from build123d import *

# Parameters (mm, degrees)
TUBE_R            = 6.5
TUBE_R_2          = 4.5
TUBE_DEPTH        = 1
PAD001_DEPTH      = 12
CYLINDER018_R     = 4.5
CYLINDER018_DEPTH = 500
CYLINDER012_R     = 11.5
CYLINDER012_DEPTH = 1
PAD_DEPTH         = 3.5
CYLINDER011_R     = 2.25
CYLINDER011_DEPTH = 10
ARRAY002_COUNT    = 3
CYLINDER010_R     = 24.5
CYLINDER010_DEPTH = 5.5
CYLINDER013_R     = 11.5
CYLINDER013_DEPTH = 10


with BuildPart() as tube:
    # Tube → Tube (new body)
    with BuildSketch(Plane.XY.offset(35.5)):
        Circle(TUBE_R)
        Circle(TUBE_R_2, mode=Mode.SUBTRACT)
    extrude(amount=TUBE_DEPTH)


with BuildPart() as obj1:
    # Sketch001 → Pad001 (new body)
    with BuildSketch(Plane.XY):
        Polygon((7.6, 0), (3.8, 6.581793), (-3.8, 6.581793), (-7.6, 0), (-3.8, -6.581793), (3.8, -6.581793), align=None)
    extrude(amount=PAD001_DEPTH)


with BuildPart() as obj1_1:
    # Body001 placement: moved
    add(obj1.part.moved(Location((0, 0, 20))))


with BuildPart() as fusion007:
    # Cylinder018 → Cylinder018 (new body)
    with BuildSketch(Plane.XY):
        Circle(CYLINDER018_R)
    extrude(amount=CYLINDER018_DEPTH)

    # Fusion007: union obj1
    add(obj1_1.part)


with BuildPart() as cylinder012:
    # Cylinder012 → Cylinder012 (new body)
    with BuildSketch(Plane.XY.offset(20)):
        Circle(CYLINDER012_R)
    extrude(amount=CYLINDER012_DEPTH)


with BuildPart() as obj2:
    # Sketch → Pad (new body)
    with BuildSketch(Plane.XY):
        Polygon((4, 0), (2, 3.464102), (-2, 3.464102), (-4, 0), (-2, -3.464102), (2, -3.464102), align=None)
    extrude(amount=PAD_DEPTH)


with BuildPart() as obj2_1:
    # Body placement: moved
    add(obj2.part.moved(Location((19.5, 0, 22))))


with BuildPart() as array002:
    # Cylinder011 → Cylinder011 (new body)
    with BuildSketch(Plane(origin=(19.5, 0, 20), x_dir=(1, 0, 0), z_dir=(0, 0, 1))):
        Circle(CYLINDER011_R)
    extrude(amount=CYLINDER011_DEPTH)

    # Fusion003: union obj2
    add(obj2_1.part)

    # Array002: Array002 ×3 about axis
    array002_axis = Axis((0, 0, 0), (0, 0, 1))


with BuildPart() as array002_1:
    add(array002.part)
    for i in range(1, ARRAY002_COUNT):
        add(array002.part.rotate(array002_axis, i * 360 / ARRAY002_COUNT))


with BuildPart() as cut006:
    # Cylinder010 → Cylinder010 (new body)
    with BuildSketch(Plane.XY.offset(20)):
        Circle(CYLINDER010_R)
    extrude(amount=CYLINDER010_DEPTH)

    # Cut005: cut Array002
    add(array002_1.part, mode=Mode.SUBTRACT)

    # Cut006: cut Cylinder012
    add(cylinder012.part, mode=Mode.SUBTRACT)


with BuildPart() as finalplanetcarrier:
    # Cylinder013 → Cylinder013 (new body)
    with BuildSketch(Plane.XY.offset(25.5)):
        Circle(CYLINDER013_R)
    extrude(amount=CYLINDER013_DEPTH)

    # Fusion008: union Cut006
    add(cut006.part)

    # Cut008: cut Fusion007
    add(fusion007.part, mode=Mode.SUBTRACT)

    # Fusion009: union Tube
    add(tube.part)


solid = finalplanetcarrier.part
Design review of the part built by this model. Coordinates are the model's own, in mm. A direction names the side the tool comes from. Round coordinates to 2 decimals unless told otherwise and drop trailing zeros. Write each loop counter-clockwise with the first axis right and the second up, starting at its lowest first coordinate (ties: lowest second). Pieces come first, ordered by that corner, then holes. Notation, with made-up numbers: M 23,16.25 L 41,16.25 A21 ccw 41,42.25 Z; hole C 28,25.5 d2. An arc over 180 degrees is marked long. One line per item, written item: value. Start each with the question number.
1. Take a section at A-A on x = 0. State the section outline as (y, z) points, then the cut area to 3 significant figures.
2. Take a section at B-B on z = 23.5. State the section outline as (x, y) points.
3. Take a section at D-D on x = -9.75. State the section outline as (y, z) points.
4. Draft analysis for pull direction X (two halves, no side actions). For faces 1 (the face through (5, -5, 21)), 2 (the face through (-1.5, 11.4, 30.4)), 3 (the face through (-4.42, 1.54, 36.5)), 4 (the face through (20, 3.464, 24)), state which applies: pulls with the +X half, pulls with the -X half, needs draft (parallel to the pull), parting line crosses it, or undercut.
5. For faces 5 (the face through (-10, -13.423, 24)), 6 (the face through (21.646, 0.676, 20.986)), 7 (the face through (0, 6.582, 26)), list the 3-axis set-ups (+Z, -Z, +X, -X, +Y, -Y) from which the entire face can be reached by the end or side of a thin tool; tool diameter is ignored.
6. To check wall thickness, follow probe 1 along Y at (x, z) = (-0.5, 26.25); probe 2 along Z at (x, y) = (10, 9); probe 3 along X at (y, z) = (18, 25). State the ranges of each line that lie inside material, in increasing order. Write a range as from..to.
7. Clearance check with flat-ended pins moving along their axes: P1, Ø6, axis at x = 17.5, z = 27, coming from the +Y side; P2, Ø4, axis at x = 18.5, z = 24, coming from the +Y side; P3, Ø5, axis at y = -4.5, z = 29.5, coming from the -X side; P4, Ø2.5, axis at x = 19.5, y = 0, coming from the -Z side. State where each tip first meets the part, or that it passes through.
8. Take a section at C-C on y = 17.5. State the section outline as (x, z) points, then the cut area to 3 significant figures.
Computed:
1. outline: M -24.5,20 L -11.5,20 L -11.5,21 L -6.58,21 L -6.58,32 L -4.5,32 L -4.5,36.5 L -6.5,36.5 L -6.5,35.5 L -11.5,35.5 L -11.5,25.5 L -24.5,25.5 Z; M 4.5,32 L 6.58,32 L 6.58,21 L 11.5,21 L 11.5,20 L 24.5,20 L 24.5,25.5 L 11.5,25.5 L 11.5,35.5 L 6.5,35.5 L 6.5,36.5 L 4.5,36.5 Z
1. area: 304 mm²
2. outline: C 0,0 d49; hole M -13.75,-16.89 L -11.75,-20.35 L -7.75,-20.35 L -5.75,-16.89 L -7.75,-13.42 L -11.75,-13.42 Z; hole M -13.75,16.89 L -11.75,13.42 L -7.75,13.42 L -5.75,16.89 L -7.75,20.35 L -11.75,20.35 Z; hole M -7.6,0 L -3.8,-6.58 L 3.8,-6.58 L 7.6,0 L 3.8,6.58 L -3.8,6.58 Z; hole M 15.5,0 L 17.5,-3.46 L 21.5,-3.46 L 23.5,0 L 21.5,3.46 L 17.5,3.46 Z
3. outline: M -22.48,20 L -19.14,20 L -19.14,22 L -20.35,22 L -20.35,25.5 L -22.48,25.5 Z; M -14.64,20 L -6.1,20 L -6.1,21 L 6.1,21 L 6.1,20 L 14.64,20 L 14.64,22 L 13.42,22 L 13.42,25.5 L 6.1,25.5 L 6.1,35.5 L -6.1,35.5 L -6.1,25.5 L -13.42,25.5 L -13.42,22 L -14.64,22 Z; M 19.14,20 L 22.48,20 L 22.48,25.5 L 20.35,25.5 L 20.35,22 L 19.14,22 Z
4. face 1: undercut
4. face 2: parting line crosses it
4. face 3: needs draft
4. face 4: undercut
5. face 5: +Z
5. face 6: +Z, -Z
5. face 7: -Z
6. probe 1: y = -11.49..-6.58, 6.58..11.49
6. probe 2: z = 20..25.5
6. probe 3: x = -16.62..-13.11, -6.39..16.62
7. P1: stops at y = 19.45
7. P2: stops at y = 18.11
7. P3: stops at x = -11.32
7. P4: passes through
8. outline: M -17.15,20 L -11.92,20 L -11.92,22 L -13.4,22 L -13.4,25.5 L -17.15,25.5 Z; M -7.58,20 L 17.15,20 L 17.15,25.5 L -6.1,25.5 L -6.1,22 L -7.58,22 Z
8. area: 154 mm²
